Build history of the part. All positions in model axes, mm. A direction names the side the tool comes from. Give positions to 0.01 mm unless a question says otherwise; leave off trailing zeros. Order: outer loops, then holes, each group sorted by start corner. A loop starts at its lowest first (then second) coordinate and runs counter-clockwise, first axis right, second up. Notation, with made-up numbers: M -36,39 L -1,39 A3 ccw -1,44 Z; hole C 89.5,73.5 d6. An arc over 180 degrees is marked long. Use CSV: the item, a comma, the result in double quotes. Start each with the question number.
Item 1: Pin check, flat tips, straight feed: P1, Ø6.5, axis at y = -244.78, z = 17.5, coming from the +X side; P2, Ø22.5, axis at x = 960, y = -242.5, coming from the +Z side. Stop position of each tip, or through.
Item 2: Band-saw the part on B-B on x = 361. Write the cut outline in (y, z).
Item 3: Which spindle directions (+Z, -Z, +X, -X, +Y, -Y) get a long thin tool onto all of the face, cutting with end or side? Do faces 5 (the flat face through (531, -241, 0)), 6 (the flat face through (1015.673, -253, 15)). Say none if no direction does.
Item 4: Two-plate mould, pull along X, no slides. Class faces 1 (the flat face through (973, -252, 25)), 2 (the flat face through (531, 25.225, 15)), 3 (the flat face through (-60.54, -249, 15)), 4 (the flat face through (531, -489.775, 18)): pulls with the +X half, pulls with the -X half, needs draft (parallel to the pull), parting line crosses it, or undercut.
Item 5: Wall check: line 1 along Y through (x, z) = (661, 16.5); line 2 along X through (y, z) = (-101, 18.25); line 3 along Y through (x, z) = (1129.25, 17.5). Give the ranges that are in metal, low to high.
Item 6: Band-saw the part on A-A on y = -476. Write the cut outline in (x, z), plus the area to 3 significant figures.
from build123d import *

# Parameters (mm, degrees)
SKETCH_1_W          = 1200
SKETCH_1_H          = 540
EXTRUDE_1_DEPTH     = 30
SKETCH_2_W          = 1170
SKETCH_2_H          = 490
CUT_EXTRUDE_1_DEPTH = 25
SKETCH_3_R          = 4
CUT_EXTRUDE_2_DEPTH = 12000
SKETCH_4_W          = 85
SKETCH_4_H          = 75
EXTRUDE_2_DEPTH     = 20
SKETCH_5_R          = 2.5
EXTRUDE_3_DEPTH     = 5


with BuildPart() as part:
    # 草图1 → 凸台-拉伸1 (new body)
    with BuildSketch(Plane.XY):
        with Locations((539.460495659, -244.775206524)):
            Rectangle(SKETCH_1_W, SKETCH_1_H)
    extrude(amount=EXTRUDE_1_DEPTH)

    # 草图2 → 切除-拉伸1 (cut)
    with BuildSketch(Plane.XY.offset(30)):
        with Locations((539.460495659, -244.775206524)):
            Rectangle(SKETCH_2_W, SKETCH_2_H)
    extrude(amount=-CUT_EXTRUDE_1_DEPTH, mode=Mode.SUBTRACT)

    # 草图3 → 切除-拉伸2 (cut)
    with BuildSketch(Plane.ZY.offset(60.539504341)):
        with Locations(Location((17.5, -244.775206524, 0), (0, 0, 180))):
            Circle(SKETCH_3_R)
    extrude(amount=-CUT_EXTRUDE_2_DEPTH, mode=Mode.SUBTRACT)

    # 草图4 → 凸台-拉伸2 (add)
    with BuildSketch(Plane.XY.offset(5)):
        with Locations((973.172943193, -252.800296094)):
            Rectangle(SKETCH_4_W, SKETCH_4_H)
    extrude(amount=EXTRUDE_2_DEPTH)

    # 草图5 → 凸台-拉伸3 (add)
    with BuildSketch(Plane.ZY.offset(-930.672943193)):
        with Locations(Location((15.686983343, -230.168976304, 0), (0, 0, 90))):
            Circle(SKETCH_5_R)
        with Locations(Location((15.686983343, -239.791974012, 0), (0, 0, 90))):
            Circle(SKETCH_5_R)
    extrude(amount=EXTRUDE_3_DEPTH)


solid = part.part
Model answer:
1,P1,"stops at x = 1015.67"
1,P2,"stops at z = 25"
2,outline,"M -514.78,0 L 25.22,0 L 25.22,30 L 0.22,30 L 0.22,5 L -489.78,5 L -489.78,30 L -514.78,30 Z"
3,face 5,"-Z, +X, -X, +Y, -Y"
3,face 6,"+Z"
4,face 1,"undercut"
4,face 2,"needs draft"
4,face 3,"pulls with the -X half"
4,face 4,"undercut"
5,line 1,"y = -514.78 to -489.78, 0.22 to 25.22"
5,line 2,"x = -60.54 to -45.54, 1124.46 to 1139.46"
5,line 3,"y = -514.78 to -248.78, -240.78 to 25.22"
6,outline,"M -60.54,0 L 1139.46,0 L 1139.46,30 L 1124.46,30 L 1124.46,5 L -45.54,5 L -45.54,30 L -60.54,30 Z"
6,area,"6,750 mm^2"
